```python
from build123d import *

# Parameters (mm, degrees)
CUT_EXTRUDE1_DEPTH = 7


with BuildPart() as part:
    # Sketch2 → Revolve1 (revolve)
    with BuildSketch(Plane(origin=(0, 0, 0), x_dir=(0, 0, -1), z_dir=(1, 0, 0)), mode=Mode.PRIVATE) as revolve1_sk:
        with BuildLine():
            Line((-26.5, 0), (-26.5, 6.058578644))
            ThreePointArc((-26.5, 6.058578644), (-26.492387953, 6.096846987), (-26.470710678, 6.129289322))
            Line((-26.470710678, 6.129289322), (-26.129289322, 6.470710678))
            ThreePointArc((-26.129289322, 6.470710678), (-26.096846987, 6.492387953), (-26.058578644, 6.5))
            Line((-26.058578644, 6.5), (-20.241421356, 6.5))
            ThreePointArc((-20.241421356, 6.5), (-20.203153013, 6.492387953), (-20.170710678, 6.470710678))
            Line((-20.170710678, 6.470710678), (-20.029289322, 6.329289322))
            ThreePointArc((-20.029289322, 6.329289322), (-19.996846987, 6.307612047), (-19.958578644, 6.3))
            Line((-19.958578644, 6.3), (-18.6625, 6.3))
            ThreePointArc((-18.6625, 6.3), (-18.547595148, 6.252404852), (-18.5, 6.1375))
            Line((-18.5, 6.1375), (-18.5, 4.535316469))
            ThreePointArc((-18.5, 4.535316469), (-18.382842712, 4.252473757), (-18.1, 4.135316469))
            Line((-18.1, 4.135316469), (-2.747523234, 4.135316469))
            ThreePointArc((-2.747523234, 4.135316469), (-2.649506093, 4.130501196), (-2.552432912, 4.11610175))
            Line((-2.552432912, 4.11610175), (-2.065348919, 4.01921472))
            ThreePointArc((-2.065348919, 4.01921472), (-1.968275737, 4.004815273), (-1.870258597, 4))
            Line((-1.870258597, 4), (25.688101184, 4))
            Line((25.688101184, 4), (26.5, 3.188101184))
            Line((26.5, 3.188101184), (26.5, 0))
            Line((26.5, 0), (-26.5, 0))
        make_face()
    revolve(revolve1_sk.sketch.rotate(Axis((0, 0, -26.5), (0, 0, 1)), 90), axis=Axis((0, 0, -26.5), (0, 0, 1)))

    # Sketch3 → Cut-Extrude1 (cut)
    with BuildSketch(Plane.XY.offset(26.5)):
        Polygon((3, -1.732050808), (3, 1.732050808), (0, 3.464101615), (-3, 1.732050808), (-3, -1.732050808), (0, -3.464101615), align=None)
    extrude(amount=-CUT_EXTRUDE1_DEPTH, mode=Mode.SUBTRACT)

    # Cut-Extrude2 cone 1 section (through the dimple's axis) → Cut-Extrude2 (revolve, cut)
    with BuildSketch(Plane(origin=(0, 0, 26.5), x_dir=(0, -1, 0), z_dir=(1, 0, 0))):
        Polygon((0, 0), (3.723909236, 0), (0, 3.723909236), align=None)
    revolve(axis=Axis((0, 0, 26.5), (0, 0, -1)), mode=Mode.SUBTRACT)


solid = part.part
```
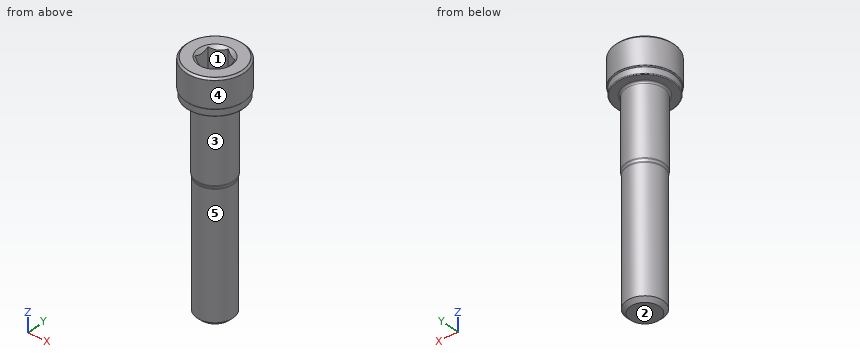
CAD build for the part. Positions are in the model's coordinates, mm. Face numbers are marked on the shaded views. A direction names the side the tool comes from. Round coordinates to 2 decimals unless told otherwise and drop trailing zeros. Order: outer loops, then holes, each group sorted by start corner. A loop starts at its lowest first (then second) coordinate and runs counter-clockwise, first axis right, second up. Notation, with made-up numbers: (-4, 73.25) - (53, 73.25) arc R28 cw to (53, 106.25) - close; hole circle Ø4 at (-15, -14). An arc over 180 degrees is marked (long way). Answer as CSV lines item,"result". Start each with the question number.
1. Pull direction X, two halves, no side cores. Call the marked faces 1, 2 and 3: +X half, -X half, draft (parallel to the pull), parting line (faces both ways), or undercut.
2. Pin check, flat tips, straight feed: pin 1 (1.5 mm diameter, centred on x = -3, z = 10.5, fed in from +Y); pin 2 (5 mm diameter, centred on y = -0.5, z = -3.5, fed in from +X); pin 3 (2 mm diameter, centred on x = 4.5, y = 1.5, fed in from -Z). Stop position of each tip, or through.
3. Drill centre lines: L1, parallel to Y at x = -0.25, z = -17; L2, parallel to Z at x = 2, y = -4.25. Where is each one in solid material? Low to high. Write a range as [from, to].
4. Saw through at A-A, the plane z = -11.5. Write the cut outline in (x, y).
5. Tool access for the marked faces 4 and 5: list every direction of +Z, -Z, +X, -X, +Y, -Y with a clear straight run to the whole face (end or side of a thin tool).
Model answer:
1,face 1,"undercut"
1,face 2,"draft"
1,face 3,"parting line"
2,pin 1,"stops at y = 3.47"
2,pin 2,"stops at x = 4"
2,pin 3,"stops at z = -25.94"
3,L1,"y = [-3.99, 3.99]"
3,L2,"z = [18.5, 26.5]"
4,outline,"circle Ø8 at (0, 0)"
5,face 4,"+Z, -Z"
5,face 5,"-Z"
